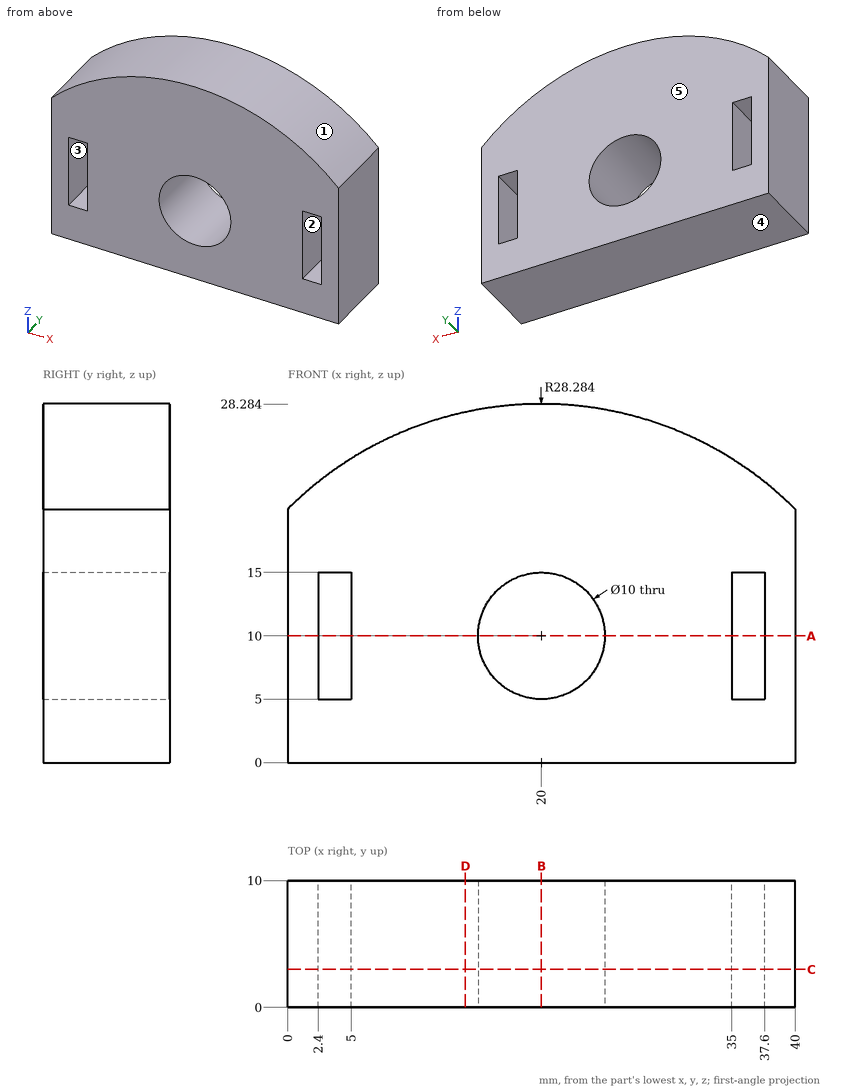
Geometry check sheet. Reference: drawing and pictorial views, mm from the part's lowest x, y, z. A direction names the side the tool comes from. Give positions to 0.01 mm unless a question says otherwise; leave off trailing zeros. Loops run counter-clockwise (first coordinate to the right, second up) from the corner with the lowest first, then second, coordinate; pieces in that order, holes last. Notation, with made-up numbers: (74.5, 3.5) - (118.5, 3.5) arc R30 cw to (118.5, 40.5) - close; hole circle Ø5 at (72, 29). An arc over 180 degrees is marked (long way). One line per question, with ' | ' between items. Start each with the question number.
1. Gauge pin test, flat ends, axial feed: pin 1 Ø0.8 at (x, y) = (36, 6.5) entering from +Z; pin 2 Ø6 at (x, y) = (12.5, 1) entering from +Z; pin 3 Ø2 at (x, y) = (3.5, 3) entering from +Z. Record the tip position at first contact, or that the pin passes through.
2. Cross-section at B-B, the plane x = 20. Enter the section's corners in (y, z).
3. Cross-section at D-D, the plane x = 14. Enter the section's corners in (y, z), plus the area to 3 significant figures.
4. Material ranges on line 1 along X through (y, z) = (5.5, 10); line 2 along X through (y, z) = (6.75, 12); line 3 along Z through (x, y) = (23.5, 7.5), recorded low to high. Write a range as [from, to].
5. Cross-section at C-C, the plane y = 3. Enter the section's corners in (x, z), plus the area to 3 significant figures.
6. Draft check along Z on the marked faces 3, 4 and 5. Enter one of: released by +Z, released by -Z, zero draft, split by the parting line, or undercut.
7. Set-up check for the marked faces 1 and 2: record each of +Z, -Z, +X, -X, +Y, -Y from which the full face is reachable in a straight line by a thin tool's end or side.
8. Cross-section at A-A, the plane z = 10. Enter the section's corners in (x, y), plus the area to 3 significant figures.
Check result:
1) pin 1: stops at z = 23.59 | pin 2: stops at z = 27.92 | pin 3: stops at z = 23.66
2) outline: (0, 0) - (10, 0) - (10, 5) - (0, 5) - close; (0, 15) - (10, 15) - (10, 28.28) - (0, 28.28) - close
3) outline: (0, 0) - (10, 0) - (10, 27.64) - (0, 27.64) - close | area: 276 mm2
4) line 1: x = [0, 2.4], [5, 15], [25, 35], [37.6, 40] | line 2: x = [0, 2.4], [5, 15.42], [24.58, 35], [37.6, 40] | line 3: z = [0, 6.43], [13.57, 28.07]
5) outline: (0, 0) - (40, 0) - (40, 20) arc R28.28 ccw to (0, 20) - close; hole (2.4, 5) - (5, 5) - (5, 15) - (2.4, 15) - close; hole circle Ø10 at (20, 10); hole (35, 5) - (37.6, 5) - (37.6, 15) - (35, 15) - close | area: 898 mm2
6) face 3: undercut | face 4: released by -Z | face 5: zero draft
7) face 1: +Z, +Y, -Y | face 2: +Y, -Y
8) outline: (0, 0) - (2.4, 0) - (2.4, 10) - (0, 10) - close; (5, 0) - (15, 0) - (15, 10) - (5, 10) - close; (25, 0) - (35, 0) - (35, 10) - (25, 10) - close; (37.6, 0) - (40, 0) - (40, 10) - (37.6, 10) - close | area: 248 mm2
